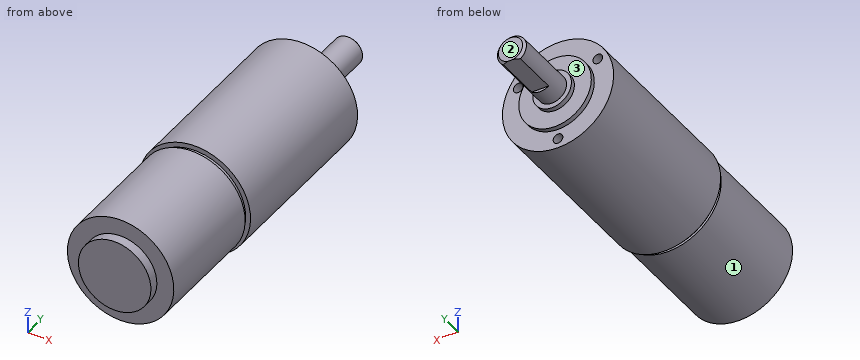
```python
from build123d import *

# Parameters (mm, degrees)
ENL_V_MAT_EXTRU_2_DEPTH = 10
CHANFREIN1_SIZE         = 0.5
ESQUISSE3_R             = 1
ENL_V_MAT_EXTRU_3_DEPTH = 4


with BuildPart() as part:
    # Esquisse1 → Révolution1 (revolve)
    with BuildSketch(Plane.XY, mode=Mode.PRIVATE) as r_volution1_sk:
        Polygon((0, 0), (7.5, 0), (7.5, 2), (11, 2), (11, 26), (10.5, 26), (10.5, 27), (11.5, 27), (11.5, 63), (7.5, 63), (7.5, 64), (4, 64), (4, 65), (3, 65), (3, 79), (0, 79), align=None)
    revolve(r_volution1_sk.sketch.rotate(Axis((0, 0, 0), (0, 1, 0)), 90), axis=Axis((0, 0, 0), (0, 1, 0)))

    # Esquisse2 → Enlèv. mat.-Extru.2 (cut)
    with BuildSketch(Plane(origin=(0, 79, 0), x_dir=(1, 0, 0), z_dir=(0, 1, 0))):
        with BuildLine():
            Line((-1.75, 2.436698586), (1.75, 2.436698586))
            ThreePointArc((1.75, 2.436698586), (0, 3), (-1.75, 2.436698586))
        make_face()
    extrude(amount=-ENL_V_MAT_EXTRU_2_DEPTH, mode=Mode.SUBTRACT)

    # Chanfrein1
    chanfrein1_edges = [part.edges().sort_by_distance(p)[0] for p in [
        (0, 79, 3),
    ]]
    chamfer(chanfrein1_edges, length=CHANFREIN1_SIZE)

    # Esquisse3 → Enlèv. mat.-Extru.3 (cut)
    with BuildSketch(Plane(origin=(0, 63, 0), x_dir=(1, 0, 0), z_dir=(0, 1, 0))):
        with Locations(Location((0, 9.5, 0), (0, 0, 270))):
            Circle(ESQUISSE3_R)
        with Locations(Location((8.227241336, -4.75, 0), (0, 0, 270))):
            Circle(ESQUISSE3_R)
        with Locations(Location((-8.227241336, -4.75, 0), (0, 0, 270))):
            Circle(ESQUISSE3_R)
    extrude(amount=-ENL_V_MAT_EXTRU_3_DEPTH, mode=Mode.SUBTRACT)


solid = part.part
```
Could you check a few things on this model? Use its own coordinates, in mm. Face numbers are marked on the shaded views. A direction names the side the tool comes from. Round coordinates to 2 decimals unless told otherwise and drop trailing zeros. Loops run counter-clockwise (first coordinate to the right, second up) from the corner with the lowest first, then second, coordinate; pieces in that order, holes last.
Q1. On a 3-axis mill with a long thin cutter (end or side, diameter ignored), from which of +Z, -Z, +X, -X, +Y, -Y can I reach the whole of each face in a straight line? I mean the marked faces 1, 2 and 3. Say none if no direction works.
Q2. I want a section at D-D (z = 9.25). Write out the boundary of the cut face in (x, y).
Q3. For P1, Ø11.5, axis at x = 5, z = -1.5, coming from the +Y side; P2, Ø5, axis at x = -8, z = -5, coming from the +Y side; P3, Ø1.5, axis at y = 40, z = 3.5, coming from the -X side; P4, Ø2.5, axis at x = 0, z = -9.5, coming from the -Y side, each with a flat end and sliding along its axis, tell me the tip position at first contact or that it passes through.
Q4. I want a section at B-B (y = 45). Write out the boundary of the cut face in (x, z).
Q5. Please list where these lines run through material, in increasing order: L1, parallel to X at y = 60.3, z = 4.75; L2, parallel to Y at x = 9.75, z = -3.25; L3, parallel to Y at x = -0.5, z = -5.
Q6. I want a section at C-C (x = 6.5). Write out the boundary of the cut face in (y, z), and give its area (3 significant figures).
Answer below:
1. face 1: -Y
1. face 2: +Z, -Z, +X, -X, +Y
1. face 3: +Y
2. outline: (-6.83, 27) - (-4.97, 27) - (-4.97, 26) - (-5.95, 26) - (-5.95, 2) - (5.95, 2) - (5.95, 26) - (4.97, 26) - (4.97, 27) - (6.83, 27) - (6.83, 63) - (-6.83, 63) - close
3. P1: stops at y = 79
3. P2: stops at y = 64
3. P3: stops at x = -11.17
3. P4: stops at y = 2
4. outline: circle Ø23 at (0, 0)
5. L1: x = -10.47 to -9.23, -7.23 to 7.23, 9.23 to 10.47
5. L2: y = 2 to 63
5. L3: y = 0 to 64
6. outline: (0, -3.74) - (2, -3.74) - (2, -8.87) - (26, -8.87) - (26, -8.25) - (27, -8.25) - (27, -9.49) - (63, -9.49) - (63, -3.74) - (64, -3.74) - (64, 3.74) - (63, 3.74) - (63, 9.49) - (27, 9.49) - (27, 8.25) - (26, 8.25) - (26, 8.87) - (2, 8.87) - (2, 3.74) - (0, 3.74) - close
6. area: 1,150 mm2
